The listing builds one solid part. Answer for the finished solid, in the listing's coordinates (mm). Coordinates: 2 decimals unless noted, no trailing zeros. Order: outer loops, then holes, each group sorted by start corner. A loop starts at its lowest first (then second) coordinate and runs counter-clockwise, first axis right, second up. Notation, with made-up numbers: (20.25, 74.5) - (36.25, 74.5) arc R32 ccw to (36.25, 110.5) - close; hole circle Ø4 at (48.5, 35.25). An arc over 180 degrees is marked (long way). Use a Markdown table: item, result. Add a question column.
Item 1: The part is cut by section B-B, the plane x = 100.5. Give the vertices of the cut face in (y, z).
Item 2: The part is cut by section A-A, the plane y = 14.5. State how many separate pieces and enclosed holes the cut face has, then the cut area to 3 significant figures.
Item 3: Find the intervals of material crossed by line 1 along Y through (x, z) = (268.5, 1.95); line 2 along Y through (x, z) = (180.5, 0.3), in increasing order.
Item 4: Flat-ended cylindrical pins translate along their axes: P1, Ø0.6, axis at y = 14.5, z = 1.5, coming from the +X side; P2, Ø1, axis at y = 15.5, z = 1, coming from the -X side. Find the tip coordinate at first contact, or state that the pin passes through.
Item 5: The mould has two halves that part along X. Classify faces 1 (the cylindrical face through (64.16, 11.75, 0.99)), 2 (the flat face through (259, 7, 2)): released by +X, released by -X, zero draft, split by the parting line, or undercut.
from build123d import *

# Parameters (mm, degrees)
EXTRUDE_1_DEPTH = 2


with BuildPart() as part:
    # Model → 凸台-拉伸1 (new body)
    with BuildSketch(Plane.XY):
        with BuildLine():
            Line((-3.696013755, 8.746558964), (49.803963076, 8.746558964))
            ThreePointArc((49.803963076, 8.746558964), (56.875030888, 11.675491152), (59.803963076, 18.746558964))
            Line((59.803963076, 18.746558964), (59.803963076, 8.746558964))
            Line((59.803963076, 8.746558964), (61.303963076, 8.746558964))
            Line((61.303963076, 8.746558964), (61.303963076, 18.746558964))
            ThreePointArc((61.303963076, 18.746558964), (64.232895264, 11.675491152), (71.303963076, 8.746558964))
            Line((71.303963076, 8.746558964), (114.803939907, 8.746558964))
            ThreePointArc((114.803939907, 8.746558964), (121.875007719, 11.675491152), (124.803939907, 18.746558964))
            Line((124.803939907, 18.746558964), (124.803939907, 8.746558964))
            Line((124.803939907, 8.746558964), (126.303939907, 8.746558964))
            Line((126.303939907, 8.746558964), (126.303939907, 18.746558964))
            ThreePointArc((126.303939907, 18.746558964), (129.232872095, 11.675491152), (136.303939907, 8.746558964))
            Line((136.303939907, 8.746558964), (179.803916738, 8.746558964))
            ThreePointArc((179.803916738, 8.746558964), (186.87498455, 11.675491152), (189.803916738, 18.746558964))
            Line((189.803916738, 18.746558964), (189.803916738, 8.746558964))
            Line((189.803916738, 8.746558964), (191.303916738, 8.746558964))
            Line((191.303916738, 8.746558964), (191.303916738, 18.746558964))
            ThreePointArc((191.303916738, 18.746558964), (194.232848927, 11.675491152), (201.303916739, 8.746558964))
            Line((201.303916739, 8.746558964), (246.003891639, 8.746558964))
            ThreePointArc((246.003891639, 8.746558964), (253.07495945, 11.675491152), (256.003891639, 18.746558964))
            Line((256.003891639, 18.746558964), (256.003891639, 8.746558964))
            Line((256.003891639, 8.746558964), (257.503891639, 8.746558964))
            Line((257.503891639, 8.746558964), (257.503891639, 18.746558964))
            ThreePointArc((257.503891639, 18.746558964), (260.432823827, 11.675491152), (267.503891639, 8.746558964))
            Line((267.503891639, 8.746558964), (275.474891639, 8.746558964))
            Line((275.474891639, 8.746558964), (292.503901751, 8.746558964))
            ThreePointArc((292.503901751, 8.746558964), (299.574969563, 11.675491152), (302.503901751, 18.746558964))
            Line((302.503901751, 18.746558964), (302.503901751, 8.746558964))
            Line((302.503901751, 8.746558964), (304.003901751, 8.746558964))
            Line((304.003901751, 8.746558964), (304.003901751, 18.746558964))
            ThreePointArc((304.003901751, 18.746558964), (306.932833939, 11.675491152), (314.003901751, 8.746558964))
            Line((314.003901751, 8.746558964), (319.003901751, 8.746558964))
            ThreePointArc((319.003901751, 8.746558964), (326.074969563, 11.675491152), (329.003901751, 18.746558964))
            Line((329.003901751, 18.746558964), (329.003901751, 8.746558964))
            Line((329.003901751, 8.746558964), (331.003901751, 8.746558964))
            Line((331.003901751, 8.746558964), (331.003901751, 18.746558964))
            ThreePointArc((331.003901751, 18.746558964), (333.932833939, 11.675491152), (341.003901751, 8.746558964))
            Line((341.003901751, 8.746558964), (358.600293959, 8.746558964))
            ThreePointArc((358.600293959, 8.746558964), (365.671361771, 11.675491152), (368.600293959, 18.746558964))
            Line((368.600293959, 18.746558964), (368.600293959, 8.746558964))
            Line((368.600293959, 8.746558964), (370.100293959, 8.746558964))
            Line((370.100293959, 8.746558964), (370.100293959, 18.746558964))
            ThreePointArc((370.100293959, 18.746558964), (373.029226147, 11.675491152), (380.10029396, 8.746558964))
            Line((380.10029396, 8.746558964), (423.600270791, 8.746558964))
            ThreePointArc((423.600270791, 8.746558964), (430.671338603, 11.675491152), (433.600270791, 18.746558964))
            Line((433.600270791, 18.746558964), (433.600270791, 8.746558964))
            Line((433.600270791, 8.746558964), (435.100270791, 8.746558964))
            Line((435.100270791, 8.746558964), (435.100270791, 18.746558964))
            ThreePointArc((435.100270791, 18.746558964), (438.029202979, 11.675491152), (445.100270791, 8.746558964))
            Line((445.100270791, 8.746558964), (488.600247622, 8.746558964))
            ThreePointArc((488.600247622, 8.746558964), (495.671315434, 11.675491152), (498.600247622, 18.746558964))
            Line((498.600247622, 18.746558964), (498.600247622, 8.746558964))
            Line((498.600247622, 8.746558964), (500.100247622, 8.746558964))
            Line((500.100247622, 8.746558964), (500.100247622, 18.746558964))
            ThreePointArc((500.100247622, 18.746558964), (503.02917981, 11.675491152), (510.100247622, 8.746558964))
            Line((510.100247622, 8.746558964), (563.600224453, 8.746558964))
            ThreePointArc((563.600224453, 8.746558964), (570.671292265, 11.675491152), (573.600224453, 18.746558964))
            Line((573.600224453, 18.746558964), (573.600224453, 8.746558964))
            Line((573.600224453, 8.746558964), (575.100224453, 8.746558964))
            Line((575.100224453, 8.746558964), (575.100224453, 3.746558964))
            Line((575.100224453, 3.746558964), (-15.196013755, 3.746558964))
            Line((-15.196013755, 3.746558964), (-15.196013755, 8.746558964))
            Line((-15.196013755, 8.746558964), (-13.696013755, 8.746558964))
            Line((-13.696013755, 8.746558964), (-13.696013755, 18.746558964))
            ThreePointArc((-13.696013755, 18.746558964), (-10.767081567, 11.675491152), (-3.696013755, 8.746558964))
        make_face()
    extrude(amount=EXTRUDE_1_DEPTH)


solid = part.part
Solution:
| question | item | result |
|---|---|---|
| 1 | outline | (3.75, 0) - (8.75, 0) - (8.75, 2) - (3.75, 2) - close |
| 2 | separate pieces | 20 |
| 2 | enclosed holes | 0 |
| 2 | area | 37.9 mm2 |
| 3 | line 1 | y = 3.75 to 8.75 |
| 3 | line 2 | y = 3.75 to 8.77 |
| 4 | P1 | stops at x = 573.6 |
| 4 | P2 | stops at x = -13.7 |
| 5 | face 1 | undercut |
| 5 | face 2 | zero draft |
